Work out the finished part from the listing and answer in its coordinate system (mm). A direction names the side the tool comes from. Round coordinates to 2 decimals unless told otherwise and drop trailing zeros. Loops run counter-clockwise (first coordinate to the right, second up) from the corner with the lowest first, then second, coordinate; pieces in that order, holes last. Notation, with made-up numbers: (-21.75, 87.25) - (13.25, 87.25) arc R6 ccw to (13.25, 98.25) - close; hole circle Ø3 at (-27, 73). An arc over 180 degrees is marked (long way). Return JSON: item names as keys, results as strings.
from build123d import *

# Parameters (mm, degrees)
F1_DEPTH  = 60.325
F2_W      = 53.0107717005
F2_H      = 22.3266
F3_DEPTH  = 44.2625842988
F4_W      = 41.91
F4_H      = 34.670740366
F5_DEPTH  = 77.503874898
F6_R      = 7.874
F7_R      = 5.08
F8_DEPTH  = 19.0500002354
F9_R      = 6.35
F10_DEPTH = 22.353


with BuildPart() as f1:
    # F0 (on Front) → F1 (new body)
    with BuildSketch(Plane.XZ):
        with BuildLine():
            Line((20.1422, -11.176), (97.1042, -11.176))
            Line((97.1042, -11.176), (97.1042, 11.176))
            Line((97.1042, 11.176), (52.9844, 11.176))
            Line((52.9844, 11.176), (52.9844, 45.974))
            Line((52.9844, 45.974), (33.9344, 45.974))
            ThreePointArc((33.9344, 45.974), (30.3602153616, 27.2583576341), (20.1422, 11.176))
            Line((20.1422, 11.176), (20.1422, -11.176))
        make_face()
        Polygon((-5.2578, -11.176), (20.1422, -11.176), (20.1422, 11.176), (-11.2522, 11.176), align=None)
        with BuildLine():
            Line((-97.1042, -11.176), (-5.2578, -11.176))
            Line((-5.2578, -11.176), (-11.2522, 11.176))
            Line((-11.2522, 11.176), (-74.7522, 11.176))
            ThreePointArc((-74.7522, 11.176), (-81.2989492269, -4.6292507731), (-97.1042, -11.176))
        make_face()
        with BuildLine():
            ThreePointArc((-74.7522, 11.176), (-112.9094507731, 26.9812507731), (-97.1042, -11.176))
            Line((-97.1042, -11.176), (-97.1042, -1.524))
            ThreePointArc((-97.1042, -1.524), (-106.0844561211, 20.1562561211), (-84.4042, 11.176))
            Line((-84.4042, 11.176), (-74.7522, 11.176))
        make_face()
        with BuildLine():
            Line((-97.1042, -1.524), (-97.1042, -11.176))
            ThreePointArc((-97.1042, -11.176), (-81.2989492269, -4.6292507731), (-74.7522, 11.176))
            Line((-74.7522, 11.176), (-84.4042, 11.176))
            ThreePointArc((-84.4042, 11.176), (-88.1239438789, 2.1957438789), (-97.1042, -1.524))
        make_face()
    extrude(amount=-F1_DEPTH)

    # F2 (on Top) → F3 (cut, symmetric)
    with BuildSketch(Plane.XY):
        with Locations((-97.226254642, 30.1625)):
            Rectangle(F2_W, F2_H)
    extrude(amount=F3_DEPTH, both=True, mode=Mode.SUBTRACT)

    # F4 (on Right) → F5 (cut)
    with BuildSketch(Plane.YZ):
        with Locations((40.005, 28.8226753473)):
            Rectangle(F4_W, F4_H)
    extrude(amount=F5_DEPTH, mode=Mode.SUBTRACT)

    # F6
    f6_edges = [f1.edges().sort_by_distance(p)[0] for p in [
        (97.1042, 30.1625, 11.176),
    ]]
    fillet(f6_edges, radius=F6_R)

    # F7
    f7_edges = [f1.edges().sort_by_distance(p)[0] for p in [
        (52.9844, 9.525, 45.974),
    ]]
    fillet(f7_edges, radius=F7_R)

    # F0 (on Front) → F8 (cut)
    with BuildSketch(Plane.XZ):
        Polygon((-5.2578, -11.176), (20.1422, -11.176), (20.1422, 11.176), (-11.2522, 11.176), align=None)
    extrude(amount=-F8_DEPTH, mode=Mode.SUBTRACT)

    # F9 (on face) → F10 (cut, through all)
    with BuildSketch(Plane.XY.offset(11.176)):
        with Locations((58.2422, 37.973)):
            Circle(F9_R)
    extrude(amount=-F10_DEPTH, mode=Mode.SUBTRACT)


solid = f1.part
1) Flat-ended cylindrical pins translate along their axes: pin 1 (10 mm diameter, centred on y = 18.5, z = 9, fed in from +X); pin 2 (10 mm diameter, centred on y = 19.5, z = 4.5, fed in from -X); pin 3 (5.5 mm diameter, centred on y = 8, z = -3.5, fed in from -X). Find the tip coordinate at first contact, or state that the pin passes through.
Verdict:
{"pin 1": "stops at x = 97.07", "pin 2": "stops at x = -119.39", "pin 3": "stops at x = -116.01"}
2) Find the intervals of material crossed by L1, parallel to X at y = 10.5, z = 15; L2, parallel to X at y = 5.5, z = 20.5; L3, parallel to Y at x = -86.5, z = 21.5 (3 decimals), in increasing order.
Verdict:
{"L1": "x = -119.13 to -109.21, -84.99 to -75.08, 23.4 to 52.98", "L2": "x = -117.42 to -105.73, -88.48 to -76.79, 27.08 to 52.98", "L3": "y = 0 to 18.999, 41.326 to 60.325"}
3) Section D-D (x = 55) is taken. Give the vertices of the cut face in (y, z) (3 decimals), and give its area (3 significant figures).
Verdict:
{"outline": "(0, -11.176) - (32.513, -11.176) - (32.513, 11.176) - (0, 11.176) - close; (43.433, -11.176) - (60.325, -11.176) - (60.325, 11.176) - (43.433, 11.176) - close", "area": "1,100 mm2"}
4) Section A-A (y = 54.5) is taken. Give the vertices of the cut face in (x, z).
Verdict:
{"outline": "(-97.1, -11.18) - (97.1, -11.18) - (97.1, 3.3) arc R7.87 ccw to (89.23, 11.18) - (52.98, 11.18) - (52.98, 11.49) - (20.43, 11.49) arc R50.8 cw to (20.14, 11.18) - (-74.75, 11.18) arc R22.35 ccw (long way) to start; hole circle Ø25.4 at (-97.1, 11.18)"}
5) Section B-B (x = -90) is taken. Give the vertices of the cut face in (y, z) (3 decimals), and give its area (3 significant figures).
Verdict:
{"outline": "(0, -11.176) - (18.999, -11.176) - (18.999, 0.649) - (0, 0.649) - close; (0, 21.703) - (18.999, 21.703) - (18.999, 32.369) - (0, 32.369) - close; (41.326, -11.176) - (60.325, -11.176) - (60.325, 0.649) - (41.326, 0.649) - close; (41.326, 21.703) - (60.325, 21.703) - (60.325, 32.369) - (41.326, 32.369) - close", "area": "855 mm2"}
6) A tool of negligible diameter and unlimited length cuts with its end or side. For faces 4 (the cylindrical face through (29.854, 9.913, 26.028)), 5 (the flat face through (-84.6, 41.326, 6.5)), 6 (the flat face through (-8.297, 9.392, 0.156)), from which of +Z, -Z, +X, -X, +Y, -Y can it reach the whole face along a straight path? Write none if from no direction.
Verdict:
{"face 4": "+Z, +Y, -Y", "face 5": "+Z, -Z, -X", "face 6": "+Z, -Y"}
7) Determine the mould class of faces 1 (the flat face through (-63, 0, 7)), 2 (the flat face through (-84.6, 18.999, 6.5)), 3 (the cylindrical face through (94.859, 30.585, 8.808)) for opening direction Y: pulls with the +Y half, pulls with the -Y half, needs draft (parallel to the pull), parting line crosses it, or undercut.
Verdict:
{"face 1": "pulls with the -Y half", "face 2": "undercut", "face 3": "needs draft"}
8) Section C-C (z = -5.5) is taken. Give the vertices of the cut face in (x, y) (3 decimals).
Verdict:
{"outline": "(-111.988, 0) - (-6.78, 0) - (-6.78, 19.05) - (20.142, 19.05) - (20.142, 0) - (97.104, 0) - (97.104, 60.325) - (-111.988, 60.325) - (-111.988, 41.326) - (-70.721, 41.326) - (-70.721, 18.999) - (-111.988, 18.999) - close; hole circle Ø12.7 at (58.242, 37.973)"}
